```python
from build123d import *

# Parameters (mm, degrees)
F0_W     = 25.4
F0_H     = 3.175
F0_W_2   = 38.1
F0_R     = 1.7859375
F0_R_2   = 0.5
F1_DEPTH = 3.175


# Not quite as in the source:
# - a length typed as a fraction of an inch, garbled in the dataset ("3 / 203.2 mm" for 3/8 in), is restored


with BuildPart() as f1:
    # F0 (on Front) → F1 (new body)
    with BuildSketch(Plane.XZ):
        with Locations((-54.5774, 81.9875024)):
            Rectangle(F0_W, F0_H)
        with Locations((16.1738, 81.9875024)):
            Rectangle(F0_W_2, F0_H)
        with Locations((86.925, 81.9875024)):
            Rectangle(F0_W, F0_H)
        with Locations((86.925, -22.7875084)):
            Rectangle(F0_W, F0_H)
        with Locations((16.1738, -22.7875084)):
            Rectangle(F0_W_2, F0_H)
        with Locations((-54.5774, -22.7875084)):
            Rectangle(F0_W, F0_H)
        Polygon((-67.2774, 57.3229712169), (-67.2774, -21.2000084), (-41.8774, -21.2000084), (-2.8762, -21.2000084), (35.2238, -21.2000084), (74.225, -21.2000084), (99.625, -21.2000084), (99.625, 80.4000024), (74.225, 80.4000024), (35.2238, 80.4000024), (-2.8762, 80.4000024), (-41.8774, 80.4000024), (-67.2774, 80.4000024), align=None)
        with Locations((-63.3824, 0)):
            Circle(F0_R, mode=Mode.SUBTRACT)
        with Locations((-55.4124, 0)):
            Circle(F0_R, mode=Mode.SUBTRACT)
        with Locations((-47.4424, 0)):
            Circle(F0_R, mode=Mode.SUBTRACT)
        with Locations((-39.4724, 0)):
            Circle(F0_R, mode=Mode.SUBTRACT)
        with Locations((-31.7, 0)):
            Circle(F0_R, mode=Mode.SUBTRACT)
        with Locations((-23.73, 0)):
            Circle(F0_R, mode=Mode.SUBTRACT)
        with Locations((-15.76, 0)):
            Circle(F0_R, mode=Mode.SUBTRACT)
        with Locations((-7.79, 0)):
            Circle(F0_R, mode=Mode.SUBTRACT)
        Circle(F0_R, mode=Mode.SUBTRACT)
        with Locations((7.97, 0)):
            Circle(F0_R, mode=Mode.SUBTRACT)
        with Locations((15.94, 0)):
            Circle(F0_R, mode=Mode.SUBTRACT)
        with Locations((23.91, 0)):
            Circle(F0_R, mode=Mode.SUBTRACT)
        with Locations((31.88, 0)):
            Circle(F0_R, mode=Mode.SUBTRACT)
        with Locations((39.85, 0)):
            Circle(F0_R, mode=Mode.SUBTRACT)
        with Locations((47.82, 0)):
            Circle(F0_R, mode=Mode.SUBTRACT)
        with Locations((55.79, 0)):
            Circle(F0_R, mode=Mode.SUBTRACT)
        with Locations((63.76, 0)):
            Circle(F0_R, mode=Mode.SUBTRACT)
        with Locations((71.73, 0)):
            Circle(F0_R, mode=Mode.SUBTRACT)
        with Locations((79.7, 0)):
            Circle(F0_R, mode=Mode.SUBTRACT)
        with Locations((87.67, 0)):
            Circle(F0_R, mode=Mode.SUBTRACT)
        with Locations((95.64, 0)):
            Circle(F0_R, mode=Mode.SUBTRACT)
        with Locations((6.74, 40.005)):
            Circle(F0_R_2, mode=Mode.SUBTRACT)
        Polygon((9.64, 40.005), (9.64, 46.305), (15.94, 46.305), (32.84, 46.305), (32.84, 33.705), (15.94, 33.705), (9.64, 33.705), align=None, mode=Mode.SUBTRACT)
        with Locations((35.74, 40.005)):
            Circle(F0_R_2, mode=Mode.SUBTRACT)
    extrude(amount=F1_DEPTH)


solid = f1.part
```
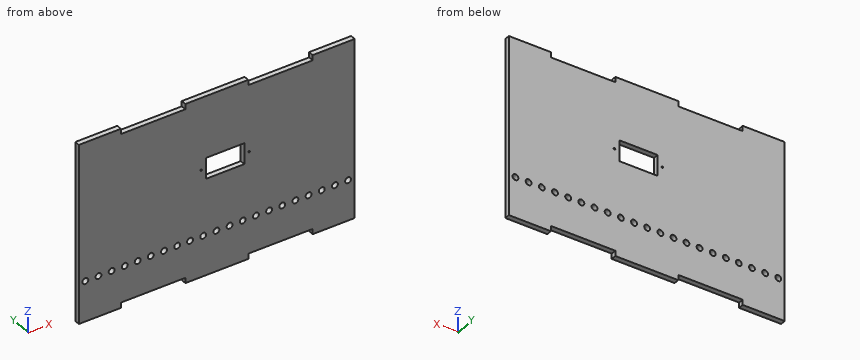
Input: part model. Units: mm. Frame: model coordinates. Give positions to 0.01 mm unless a question says otherwise; leave off trailing zeros. Order: outer loops, then holes, each group sorted by start corner. A loop starts at its lowest first (then second) coordinate and runs counter-clockwise, first axis right, second up. Notation, with made-up numbers: M 85.25,5.25 L 125.25,5.25 A27 ccw 125.25,43.25 Z; hole C 17.5,33 d8. An arc over 180 degrees is marked long. One line per question, with ' | ' between items. Start each with the question number.
1. Section query B-B (x = 71.73). Return the cut outline in (y, z) (3 decimals).
2. Section query C-C (y = -0.7). Count the separate pieces of the cut face and the enclosed holes in it, and give its area (3 significant figures).
3. Section query D-D (x = -35.5). Return the cut outline in (y, z) (3 decimals).
4. Material intervals for probe 1 along Z at (x, y) = (20, -1.7) (3 decimals); probe 2 along Z at (x, y) = (95.64, -1.9) (3 decimals); probe 3 along Z at (x, y) = (44, -3), sorted ascending. Write a range as [from, to].
5. Section query A-A (x = 15.94). Return the cut outline in (y, z) (3 decimals).
6. First-contact query: pin 1 Ø1 at (x, y) = (-40, -0.5) entering from +Z. Flat tip, straight axial feed; report the tip coordinate or a pass-through.
Here are the results:
1) outline: M -3.175,-21.2 L 0,-21.2 L 0,-1.786 L -3.175,-1.786 Z; M -3.175,1.786 L 0,1.786 L 0,80.4 L -3.175,80.4 Z
2) separate pieces: 1 | enclosed holes: 24 | area: 17,000 mm²
3) outline: M -3.175,-21.2 L 0,-21.2 L 0,80.4 L -3.175,80.4 Z
4) probe 1: [-24.375, 33.705], [46.305, 83.575] | probe 2: [-24.375, -1.786], [1.786, 83.575] | probe 3: [-21.2, 80.4]
5) outline: M -3.175,-24.375 L 0,-24.375 L 0,-1.786 L -3.175,-1.786 Z; M -3.175,1.786 L 0,1.786 L 0,33.705 L -3.175,33.705 Z; M -3.175,46.305 L 0,46.305 L 0,83.575 L -3.175,83.575 Z
6) pin 1: z = 80.4
